Autodesk Fusion 360 part; units mm, degrees
sketch "Sketch1" plane through (0, 0, 69) normal (0, 0, 1) x (-1, 0, 0)
  circle A0 centre (29.17, 30.575) radius 3.05
  circle A1 centre (70.83, 30.575) radius 3.05
  line L0 (24.17, 21.15) -> (75.83, 21.15)
  line L1 (75.83, 21.15) -> (75.83, 30.575)
  arc A2 (75.83, 30.575) -> (70.83, 35.575) centre (70.83, 30.575) ccw
  line L2 (70.83, 35.575) -> (29.17, 35.575)
  arc A3 (29.17, 35.575) -> (24.17, 30.575) centre (29.17, 30.575) ccw
  line L3 (24.17, 30.575) -> (24.17, 21.15)
  line L4 (29.8595, -5) -> (27.8595, -5)
  arc A4 (23.8595, -1) -> (27.8595, -5) centre (27.8595, -1) ccw
  line L5 (23.8595, -1) -> (23.8595, 1)
  arc A5 (27.8595, 5) -> (23.8595, 1) centre (27.8595, 1) ccw
  line L6 (27.8595, 5) -> (29.8595, 5)
  arc A6 (33.8595, 1) -> (29.8595, 5) centre (29.8595, 1) ccw
  line L7 (33.8595, 1) -> (33.8595, -1)
  arc A7 (29.8595, -5) -> (33.8595, -1) centre (29.8595, -1) ccw
  circle A8 centre (50, 0) radius 10
  line L8 (76.1405, 1) -> (76.1405, -1)
  arc A9 (72.1405, -5) -> (76.1405, -1) centre (72.1405, -1) ccw
  line L9 (72.1405, -5) -> (70.1405, -5)
  arc A10 (66.1405, -1) -> (70.1405, -5) centre (70.1405, -1) ccw
  line L10 (66.1405, -1) -> (66.1405, 1)
  arc A11 (70.1405, 5) -> (66.1405, 1) centre (70.1405, 1) ccw
  line L11 (70.1405, 5) -> (72.1405, 5)
  arc A12 (76.1405, 1) -> (72.1405, 5) centre (72.1405, 1) ccw
  circle A13 centre (95.6212, 10.575) radius 1.5
  circle A14 centre (37.085, 10.575) radius 1.5
  circle A15 centre (62.915, 10.575) radius 1.5
  circle A16 centre (37.085, -10.575) radius 1.5
  circle A17 centre (62.915, -10.575) radius 1.5
  circle A18 centre (4.3788, 10.575) radius 1.5
  circle A19 centre (95.6212, -10.575) radius 1.5
  circle A20 centre (4.3788, -10.575) radius 1.5
  line L12 (-10, -21.15) -> (110, -21.15)
  line L13 (110, -21.15) -> (110, 21.15)
  line L14 (110, 21.15) -> (-10, 21.15)
  line L15 (-10, 21.15) -> (-10, -21.15)
  line L16 (24.17, 21.55) -> (75.83, 21.55)
  dimension "d176" = -0.4
extrude "Extrude1" add sketch "Sketch1" along normal blind 2 contours L1 A2 L2 A3 L3 L16
sketch "Sketch2" plane through (0, -35.575, 0) normal (0, -1, 0) x (1, 0, 0)
  line L0 (-70.83, 69) -> (-29.17, 69)
  line L1 (-29.17, 69) -> (-29.17, 71)
  line L2 (-29.17, 71) -> (-70.83, 71)
  line L3 (-70.83, 71) -> (-70.83, 69)
  line L4 (9.9999, 77.6216) -> (10, 92) construction
  line L5 (10, 92) -> (-110, 92) construction
  line L6 (-110, 92) -> (-109.9999, 77.6216) construction
  line L7 (-109.9999, 77.6216) -> (-98.6213, 89) construction
  line L8 (-98.6213, 89) -> (-92.6213, 89) construction
  line L9 (-92.6213, 89) -> (-81.2425, 77.621) construction
  line L10 (-81.2425, 77.621) -> (-81.2425, 89) construction
  line L11 (-81.2425, 89) -> (-18.7575, 89) construction
  line L12 (-18.7575, 89) -> (-18.7575, 77.621) construction
  line L13 (-18.7575, 77.621) -> (-7.3788, 89) construction
  line L14 (-7.3788, 89) -> (-1.3788, 89) construction
  line L15 (-1.3788, 89) -> (9.9999, 77.6216) construction
  line L16 (-50, 70) -> (-50, 89)
  circle A0 centre (-50, 79.5) radius 10.5
  arc A1 (-40.8349, 71) -> (-59.1652, 71) centre (-50, 79.5) ccw
  line L17 (-59.1652, 71) -> (-70.83, 71) construction
  line L18 (-40.8349, 71) -> (-29.17, 71) construction
  line L19 (-64.9976, 71) -> (-62.1298, 82.5197)
  line L20 (-35.0024, 71) -> (-37.8702, 82.5197)
  dimension "d179" = 21
extrude "Extrude2" add sketch "Sketch2" against normal blind 14.025 contours L2 A0 A1 | L2 A1 L19 | L2 A1 L20
sketch "Sketch3" plane through (0, -35.575, 0) normal (0, -1, 0) x (1, 0, 0)
  line L0 (-64.9976, 71) -> (-70.83, 71)
  line L1 (-70.83, 71) -> (-70.83, 69)
  line L2 (-70.83, 69) -> (-29.17, 69)
  line L3 (-29.17, 69) -> (-29.17, 71)
  line L4 (-29.17, 71) -> (-35.0024, 71)
  line L5 (-35.0024, 71) -> (-37.8702, 82.5197)
  arc A0 (-37.8702, 82.5197) -> (-62.1298, 82.5197) centre (-50, 79.5) ccw
  line L6 (-62.1298, 82.5197) -> (-64.9976, 71)
  arc A1 (-43.8356, 71) -> (-56.1644, 71) centre (-50, 79.5) ccw
  line L7 (-43.8356, 71) -> (-56.1644, 71)
  line L8 (-59.1687, 74.3828) -> (-56.1644, 69)
  line L9 (-50, 69) -> (-50, 90) construction
  line L10 (-40.8313, 74.3828) -> (-43.8356, 69)
  arc A2 (-40.8313, 74.3828) -> (-59.1687, 74.3828) centre (-50, 79.5) ccw
  dimension "d183" = 21
extrude "Extrude3" cut sketch "Sketch3" against normal blind 14.025 contours L2 A1 L7 L8 L10
sketch "Sketch4" plane through (0, 0, 71) normal (0, 0, 1) x (-1, 0, 0)
  line L0 (64.9976, 35.575) -> (64.9976, 21.55)
  line L1 (64.9976, 21.55) -> (75.83, 21.55)
  line L2 (75.83, 21.55) -> (75.83, 30.575)
  arc A0 (75.83, 30.575) -> (70.83, 35.575) centre (70.83, 30.575) ccw
  line L3 (70.83, 35.575) -> (64.9976, 35.575)
  circle A1 centre (70.83, 30.575) radius 3.05
  line L4 (62.1298, 35.575) -> (37.8702, 35.575)
  line L5 (37.8702, 35.575) -> (37.8702, 21.55)
  line L6 (37.8702, 21.55) -> (62.1298, 21.55)
  line L7 (62.1298, 21.55) -> (62.1298, 35.575)
  line L8 (64.9976, 35.575) -> (62.1298, 35.575)
  line L9 (62.1298, 35.575) -> (62.1298, 21.55)
  line L10 (62.1298, 21.55) -> (64.9976, 21.55)
  line L11 (64.9976, 21.55) -> (64.9976, 35.575)
  line L12 (37.8702, 35.575) -> (35.0024, 35.575)
  line L13 (35.0024, 35.575) -> (35.0024, 21.55)
  line L14 (35.0024, 21.55) -> (37.8702, 21.55)
  line L15 (37.8702, 21.55) -> (37.8702, 35.575)
  circle A2 centre (29.17, 30.575) radius 3.05
  line L16 (35.0024, 21.55) -> (35.0024, 35.575)
  line L17 (35.0024, 35.575) -> (29.17, 35.575)
  arc A3 (29.17, 35.575) -> (24.17, 30.575) centre (29.17, 30.575) ccw
  line L18 (24.17, 30.575) -> (24.17, 21.55)
  line L19 (24.17, 21.55) -> (35.0024, 21.55)
  line L20 (50, 21.55) -> (50, 35.575) construction
  circle A4 centre (70.83, 30.575) radius 1.5
  circle A5 centre (29.17, 30.575) radius 1.5
  dimension "d186" = 3
  dimension "d187" = 3
extrude "Extrude4" add sketch "Sketch4" against normal blind 2 contours A1 | A2
delete_face "DeleteFace1" 1 faces at (-75.1601, -33.075, 70.3333)
delete_face "DeleteFace2" 1 faces at (-24.445, -32.2103, 70.3333)
sketch "Sketch5" plane through (0, -35.575, 0) normal (0, -1, 0) x (1, 0, 0)
  line L0 (-24.17, 71) -> (-35.0024, 71)
  line L1 (-35.0024, 71) -> (-37.8702, 82.5197)
  arc A0 (-37.8702, 82.5197) -> (-62.1298, 82.5197) centre (-50, 79.5) ccw
  line L2 (-62.1298, 82.5197) -> (-64.9976, 71)
  line L3 (-64.9976, 71) -> (-75.83, 71)
  line L4 (-75.83, 71) -> (-75.83, 69)
  line L5 (-75.83, 69) -> (-56.1644, 69)
  line L6 (-56.1644, 69) -> (-59.1687, 74.3828)
  arc A1 (-40.8313, 74.3828) -> (-59.1687, 74.3828) centre (-50, 79.5) ccw
  line L7 (-40.8313, 74.3828) -> (-43.8356, 69)
  line L8 (-43.8356, 69) -> (-24.17, 69)
  line L9 (-24.17, 69) -> (-24.17, 71)
  line L10 (-70.4138, 71) -> (-70.4138, 80) construction
  line L11 (-50, 92) -> (-50, 68.7831) construction
  line L12 (-75.83, 71) -> (-75.83, 80)
  line L13 (-75.83, 80) -> (-62.7571, 80)
  line L14 (-24.17, 71) -> (-24.17, 80)
  line L15 (-24.17, 80) -> (-37.243, 80)
  dimension "d297" = 9
extrude "Extrude5" add sketch "Sketch5" against normal blind 14.025 contours L0 L1 L14 L15 | L2 L3 L12 L13
extrude "Extrude6" cut 2 faces at (-70.0515, -30.2933, 71) (-28.7569, -30.8567, 71) along direction (0, 0, 1) blind 9
fillet "Fillet1" radius 5 5 edges at (-75.83, -35.575, 74.5) (-24.17, -35.575, 75.5) (-24.17, -35.575, 70) (-24.17, -35.575, 75.5) (-24.17, -35.575, 70)
fillet "Fillet2" radius 3 8 edges at (-69.2935, -21.55, 80) (-66.7935, -35.575, 80) (-74.3655, -34.1105, 80) (-75.83, -26.0625, 80) (-30.7065, -21.55, 80) (-33.2065, -35.575, 80) (-25.6345, -34.1105, 80) (-24.17, -26.0625, 80)
Work out the finished part from the listing and answer in its coordinate system (mm). A direction names the side the tool comes from. Coordinates: 2 decimals unless noted, no trailing zeros. Write each loop counter-clockwise with the first axis right and the second up, starting at its lowest first coordinate (ties: lowest second). Pieces come first, ordered by that corner, then holes.
1. Consider line 1 along Y through (x, z) = (-29.17, 72.25) (3 decimals); line 2 along Z through (x, y) = (-50, -28.5); line 3 along X through (y, z) = (-23, 71.75). Determine where each line is inside the solid, lowest interval first.
Results list:
line 1: y = -35.575 to -32.075, -29.075 to -21.55
line 2: z = 90 to 92
line 3: x = -75.83 to -57.7, -42.3 to -24.17
2. The part is cut by section C-C, the plane z = 76. State how many separate pieces and enclosed holes the cut face has, and give its area (3 significant figures).
Results list:
separate pieces: 2
enclosed holes: 2
area: 422 mm2
3. The part is cut by section D-D, the plane y = -28.5. Write down the section's boundary in (x, z), and give its area (3 significant figures).
Results list:
outline: (-75.83, 69) - (-56.16, 69) - (-59.17, 74.38) arc R10.5 cw (long way) to (-40.83, 74.38) - (-43.84, 69) - (-24.17, 69) - (-24.17, 77) arc R3 ccw to (-27.17, 80) - (-37.24, 80) - (-37.87, 82.52) arc R12.5 ccw to (-62.13, 82.52) - (-62.76, 80) - (-72.83, 80) arc R3 ccw to (-75.83, 77) - close
area: 439 mm2
4. Flat-ended cylindrical pins translate along their axes: pin 1 (5 mm diameter, centred on x = -70.5, y = -30.5, fed in from +Z); pin 2 (8 mm diameter, centred on x = -47, z = 81.5, fed in from +Y); pin 3 (8 mm diameter, centred on y = -32.5, z = 85, fed in from +X); pin 4 (4 mm diameter, centred on y = -27, z = 88, fed in from +X). Find the tip coordinate at first contact, or state that the pin passes through.
Results list:
pin 1: stops at z = 80
pin 2: passes through
pin 3: stops at x = -37.49
pin 4: stops at x = -39.32
5. For a pull along X with two mould halves and no side action, classify faces 1 (the cylindrical face through (-69.724, -29.561, 74.423)), 2 (the flat face through (-32, -29, 80)), 3 (the cylindrical face through (-25.596, -34.071, 72.944)), 4 (the flat face through (-62.52, -28.66, 80.95)) as +X half, -X half, draft (parallel to the pull), parting line (faces both ways), or undercut.
Results list:
face 1: undercut
face 2: draft
face 3: +X half
face 4: -X half
6. The part is cut by section B-B, the plane z = 83.25. Write down the section's boundary in (x, y) (3 decimals).
Results list:
outline: (-61.924, -35.575) - (-59.808, -35.575) - (-59.808, -21.55) - (-61.924, -21.55) - close; (-40.192, -35.575) - (-38.076, -35.575) - (-38.076, -21.55) - (-40.192, -21.55) - close
7. For faces 5 (the flat face through (-57.69, -28.66, 71.73)), 6 (the cylindrical face through (-69.2, -22.41, 79.1)), 7 (the cylindrical face through (-66.737, -34.673, 79.145)), determine the directions among +Z, -Z, +X, -X, +Y, -Y from which every point of the face is accessible in a straight line to the end or side of a thin tool.
Results list:
face 5: +Y, -Y
face 6: +Z, -X, +Y
face 7: +Z, -X, -Y
8. The part is cut by section A-A, the plane z = 70.75. Write down the section's boundary in (x, y) (3 decimals).
Results list:
outline: (-75.83, -30.575) arc R5 ccw to (-70.83, -35.575) - (-57.141, -35.575) - (-57.141, -21.55) - (-75.83, -21.55) - close; (-42.859, -35.575) - (-29.17, -35.575) arc R5 ccw to (-24.17, -30.575) - (-24.17, -21.55) - (-42.859, -21.55) - close; hole circle Ø3 at (-70.83, -30.575); hole circle Ø3 at (-29.17, -30.575)
